The model under review builds one solid part; all positions refer to its coordinate system, in mm. Face numbers are marked on the shaded views. A direction names the side the tool comes from. Coordinates: 2 decimals unless noted, no trailing zeros. Loops run counter-clockwise (first coordinate to the right, second up) from the corner with the lowest first, then second, coordinate; pieces in that order, holes last. Notation, with made-up numbers: M 41,24 L 91,24 A21 cw 91,42 Z; hole C 19.5,1 d7. An arc over 180 degrees is marked long. Use CSV: the item, a comma, the result in double quotes. Start each with the question number.
1. Add section D-D, the plane y = -18.5. Write out the cut boundary in (x, z), then the cut area to 3 significant figures.
2. Add section B-B, the plane z = 10.5. Write out the cut boundary in (x, y).
3. Tool access review of the marked faces 1, 2 and 3: name each direction out of +Z, -Z, +X, -X, +Y, -Y from which nothing blocks a thin tool from reaching the whole face with its end or side.
4. Add section A-A, the plane y = 0. Write out the cut boundary in (x, z), then the cut area to 3 significant figures.
5. Add section C-C, the plane x = 62.5. Write out the cut boundary in (y, z), then the cut area to 3 significant figures.
6. For L1, parallel to Z at x = 21, y = 12.5; L2, parallel to X at y = 16, z = 9.5; L3, parallel to Y at x = 54.5, z = 19, list the stretches that pass through material, from the lowest coordinate up.
7. Draft analysis for pull direction Y (two halves, no side actions). For the marked faces 4, 5, 6 and 7, state which applies: +Y half, -Y half, draft (parallel to the pull), parting line (faces both ways), or undercut.
8. Clearance check with flat-ended pins moving along their axes: P1, Ø6.5, axis at x = 8, z = 8.5, coming from the +Y side; P2, Ø12, axis at x = -13.5, y = 18.5, coming from the +Z side; P3, Ø3, axis at x = -13.5, y = 22.5, coming from the -Z side; P4, Ø2, axis at y = 1, z = 24, coming from the -X side. State where each tip first meets the part, or that it passes through.
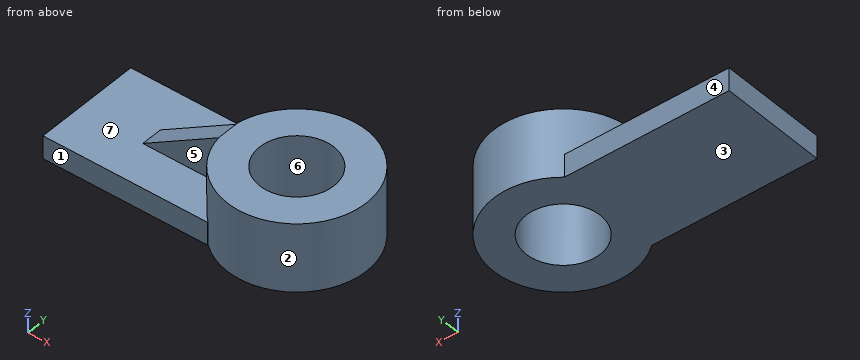
from build123d import *

# Parameters (mm, degrees)
F1_DEPTH = 12.7
F2_R     = 38.728544
F3_DEPTH = 38.1
F4_W     = 42.172854
F4_H     = 11.782876
F5_DEPTH = 25.4
F7_DEPTH = 25.4
F8_R     = 20.660809
F9_DEPTH = 50.8


with BuildPart() as f1:
    # F0 (on Top) → F1 (new body)
    with BuildSketch(Plane.XY):
        with BuildLine():
            Line((38.757574, 29.522406), (-52.804671, 29.522406))
            Line((-52.804671, 29.522406), (-52.804671, -29.807648))
            Line((-52.804671, -29.807648), (38.757574, -29.807648))
            Line((38.757574, -29.807648), (38.757574, -29.413341))
            ThreePointArc((38.757574, -29.413341), (26.480182, 0), (38.757574, 29.413341))
            Line((38.757574, 29.413341), (38.757574, 29.522406))
        make_face()
    extrude(amount=F1_DEPTH)

    # F2 (on Top) → F3 (join)
    with BuildSketch(Plane.XY):
        with Locations((63.900545, 0)):
            Circle(F2_R)
    extrude(amount=F3_DEPTH)

    # F4 (on face) → F5 (join)
    with BuildSketch(Plane.XY.offset(12.7)):
        with Locations((4.635942, -0.614486)):
            Rectangle(F4_W, F4_H)
    extrude(amount=F5_DEPTH)

    # F6 (on face) → F7 (cut)
    with BuildSketch(Plane.XZ.offset(6.505924)):
        Polygon((-16.450485, 12.7), (25.722369, 38.1), (-16.450485, 38.1), align=None)
    extrude(amount=-F7_DEPTH, mode=Mode.SUBTRACT)

    # F8 (on face) → F9 (cut)
    with BuildSketch(Plane.XY.offset(38.1)):
        with Locations((63.900545, 0)):
            Circle(F8_R)
    extrude(amount=-F9_DEPTH, mode=Mode.SUBTRACT)


solid = f1.part
Computed:
1,outline,"M -52.8,0 L 54.7,0 L 54.7,38.1 L 29.88,38.1 L 29.88,12.7 L -52.8,12.7 Z; M 73.1,0 L 97.92,0 L 97.92,38.1 L 73.1,38.1 Z"
1,area,"2,940 mm^2"
2,outline,"M -52.8,-29.81 L 38.76,-29.81 L 38.76,-29.46 A38.73 ccw long 38.76,29.46 L 38.76,29.52 L -52.8,29.52 Z; hole C 63.9,0 d41.32"
3,face 1,"+Z, -Z, -X, -Y"
3,face 2,"+Z"
3,face 3,"-Z, +X, -X, +Y, -Y"
4,outline,"M -52.8,0 L 43.24,0 L 43.24,38.1 L 25.72,38.1 L -16.45,12.7 L -52.8,12.7 Z; M 84.56,0 L 102.63,0 L 102.63,38.1 L 84.56,38.1 Z"
4,area,"2,890 mm^2"
5,outline,"M -38.7,0 L -20.61,0 L -20.61,38.1 L -38.7,38.1 Z; M 20.61,0 L 38.7,0 L 38.7,38.1 L 20.61,38.1 Z"
5,area,"1,380 mm^2"
6,L1,"z = 0 to 12.7"
6,L2,"x = -52.8 to 50.83, 76.97 to 99.17"
6,L3,"y = -37.57 to -18.4, 18.4 to 37.57"
7,face 4,"+Y half"
7,face 5,"-Y half"
7,face 6,"undercut"
7,face 7,"draft"
8,P1,"stops at y = 29.52"
8,P2,"stops at z = 12.7"
8,P3,"stops at z = 0"
8,P4,"stops at x = 0.65"
